Work out the finished part from the listing and answer in its coordinate system (mm). A direction names the side the tool comes from. Round coordinates to 2 decimals unless told otherwise and drop trailing zeros. Loops run counter-clockwise (first coordinate to the right, second up) from the corner with the lowest first, then second, coordinate; pieces in that order, holes last.
Autodesk Inventor part; units mm, degrees
ref_plane "YZ Plane" through (0, 0, 0) normal (1, 0, 0) x (0, 1, 0)
ref_plane "XZ Plane" through (0, 0, 0) normal (0, 1, 0) x (-1, 0, 0)
ref_plane "XY Plane" through (0, 0, 0) normal (0, 0, 1) x (1, 0, 0)
sketch "Sketch1" plane through (0, 0, 0) normal (0, 0, 1) x (1, 0, 0)
  line L0 (-12.7, -25.4) -> (12.7, -25.4)
  line L1 (12.7, -25.4) -> (12.7, 25.4)
  line L2 (12.7, 25.4) -> (-12.7, 25.4)
  line L3 (-12.7, 25.4) -> (-12.7, -25.4)
  line L4 (-12.7, -25.4) -> (12.7, 25.4) construction
  line L5 (12.7, -25.4) -> (-12.7, 25.4) construction
  line L6 (-10.16, -22.86) -> (10.16, -22.86)
  line L7 (10.16, -22.86) -> (10.16, 22.86)
  line L8 (10.16, 22.86) -> (-10.16, 22.86)
  line L9 (-10.16, 22.86) -> (-10.16, -22.86)
  line L10 (-10.16, -22.86) -> (10.16, 22.86) construction
  line L11 (10.16, -22.86) -> (-10.16, 22.86) construction
  point P0 (0, 0)
  dimension "d0" = 25.4
  dimension "d1" = 50.8
  dimension "d2" = 20.32
  dimension "d3" = 45.72
extrude "Extrusion1" add sketch "Sketch1" along normal mid plane 279.4
sketch "Sketch2" plane through (-12.7, 25.4, 139.7) normal (0, 1, 0) x (1, 0, 0)
  line L0 (25.4, 279.4) -> (25.4, 0)
  line L1 (25.4, 0) -> (0, 0)
  point P0 (12.7, 139.7)
  point P1 (12.7, 12.7)
  dimension "d6" = 12.7
  dimension "d7" = 12.7
hole "Hole1" at (0, 25.4, 127) direction (0, -1, 0) diameter 4.1402 end through all
pattern_linear "Rectangular Pattern1" count 11 spacing 25.4 along (0, 0, -1) of "Hole1"
sketch "Sketch3" plane through (-12.7, -25.4, 139.7) normal (-1, 0, 0) x (0, 0, 1)
  line L0 (0, 0) -> (-279.4, 0)
  line L1 (0, 50.8) -> (0, 0)
  point P0 (-139.7, 25.4)
  point P1 (-12.7, 12.7)
  dimension "d18" = 12.7
  dimension "d19" = 12.7
hole "Hole2" at (-12.7, -12.7, 127) direction (1, 0, 0) diameter 4.1402 end through all
properties part number "Outtake_vertical_frame"
1. Determine the mould class of faces 3 (the face through (2, -22.86, -2)), 4 (the face through (3, -25.4, -2)), 5 (the face through (-3, 25.4, -2)), 6 (the face through (-10.4, 2, 139.7)) for opening direction Y: +Y half, -Y half, draft (parallel to the pull), parting line (faces both ways), or undercut.
Answer key:
face 3: undercut
face 4: -Y half
face 5: +Y half
face 6: draft
2. Consider probe 1 along Y at (x, z) = (-1.25, 107.5); probe 2 along X at (y, z) = (-13, -8.5); probe 3 along X at (y, z) = (24.1, 76.2). Determine where each line is inside the solid, lowest interval first.
Answer key:
probe 1: y = -25.4 to -22.86, 22.86 to 25.4
probe 2: x = -12.7 to -10.16, 10.16 to 12.7
probe 3: x = -12.7 to -2.07, 2.07 to 12.7
3. Find section B-B (x = -6.75). Write down the section's boundary in (y, z), then the cut area to 3 significant figures.
Answer key:
outline: (-25.4, -139.7) - (-22.86, -139.7) - (-22.86, 139.7) - (-25.4, 139.7) - close; (22.86, -139.7) - (25.4, -139.7) - (25.4, 139.7) - (22.86, 139.7) - close
area: 1,420 mm2
4. Find section A-A (y = 19.5). Write down the section's boundary in (x, z), then the cut area to 3 significant figures.
Answer key:
outline: (-12.7, -139.7) - (-10.16, -139.7) - (-10.16, 139.7) - (-12.7, 139.7) - close; (10.16, -139.7) - (12.7, -139.7) - (12.7, 139.7) - (10.16, 139.7) - close
area: 1,420 mm2
5. Which of the six approach directions +Z, -Z, +X, -X, +Y, -Y give full straight-line access (tool end or side, diameter ignored) to faces 1 (the face through (10.16, 0, -2)), 2 (the face through (-10.4, 2, -139.7))?
Answer key:
face 1: +Z, -Z
face 2: -Z, +X, -X, +Y, -Y
6. Given pin 1 (2.5 mm diameter, centred on x = 0, z = 127, fed in from -Y), flat-ended and moving along its own axis, determine where the tip first touches the part or whether it passes through.
Answer key:
pin 1: passes through
7. Find section C-C (z = 15). Write down the section's boundary in (x, y).
Answer key:
outline: (-12.7, -25.4) - (12.7, -25.4) - (12.7, 25.4) - (-12.7, 25.4) - close; hole (-10.16, -22.86) - (10.16, -22.86) - (10.16, 22.86) - (-10.16, 22.86) - close
